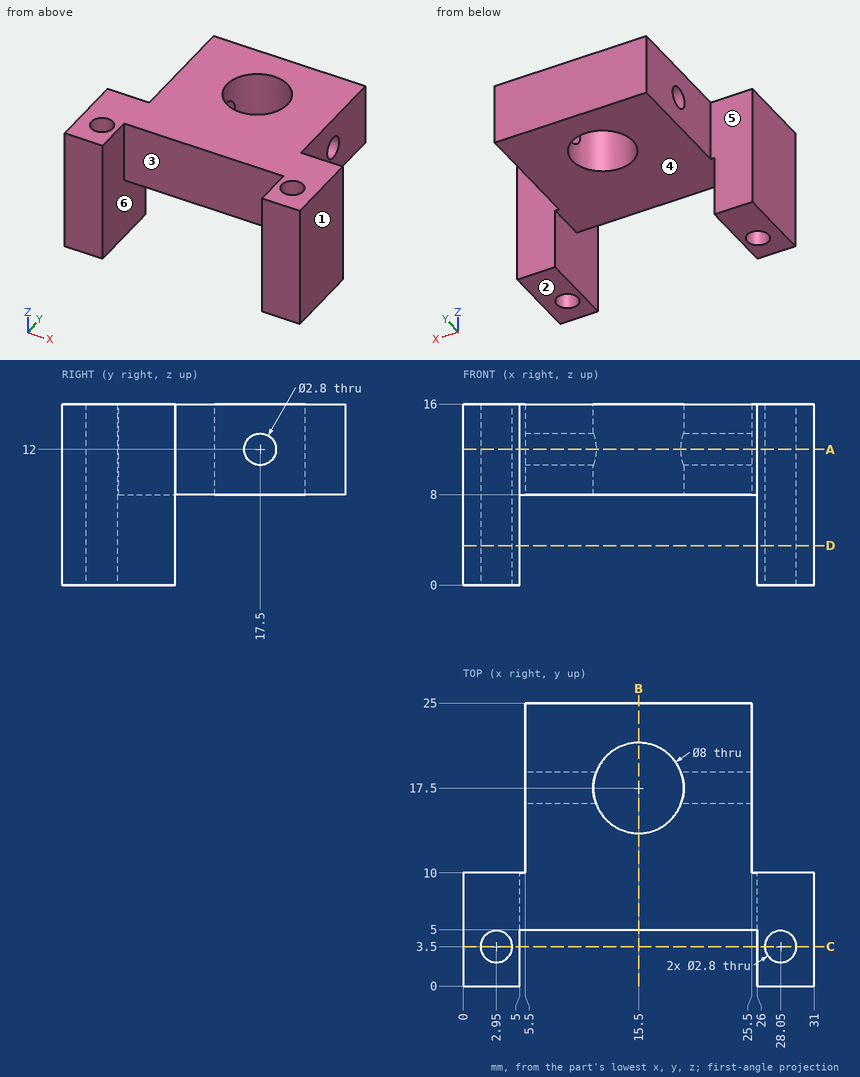
For this review, use the dimensioned drawing (mm, ordinates from the lowest corner) and the shaded views. A direction names the side the tool comes from. Coordinates: 2 decimals unless noted, no trailing zeros. Order: outer loops, then holes, each group sorted by start corner. A loop starts at its lowest first (then second) coordinate and runs counter-clockwise, first axis right, second up. Notation, with made-up numbers: (-16.5, 39.5) -> (37.5, 39.5) arc R10 ccw to (37.5, 48.5) -> close; hole circle Ø8 at (-24, -14.5). An arc over 180 degrees is marked (long way). One line per item, written item: value. Start each with the question number.
Q1. Take a section at B-B, the plane x = 15.5. State the section outline as (y, z) points.
Q2. Take a section at A-A, the plane z = 12. State the section outline as (x, y) points, then the cut area to 3 significant figures.
Q3. Tool access review of the marked faces 4, 5 and 6: name each direction out of +Z, -Z, +X, -X, +Y, -Y from which nothing blocks a thin tool from reaching the whole face with its end or side.
Q4. Insertion check: pin 1 Ø3 at (x, z) = (2.5, 11.5) entering from +Y; pin 2 Ø3 at (x, z) = (12, 12.5) entering from -Y; pin 3 Ø2.5 at (y, z) = (17.5, 11.5) entering from -X. Each pin has a flat end and moves straight along its axis. Give the tip position at first contact, or say it passes through.
Q5. For probe 1 along Y at (x, z) = (24.25, 12); probe 2 along X at (y, z) = (4.5, 12.5); probe 3 along Y at (x, z) = (15.5, 13), list the stretches that pass through material, from the lowest coordinate up.
Q6. Mouldability with a two-part tool opening along X and no side actions: class the marked faces 1, 2 and 3 as pulls with the +X half, pulls with the -X half, needs draft (parallel to the pull), parting line crosses it, or undercut.
Q7. Take a section at D-D, the plane z = 3.5. State the section outline as (x, y) points.
Q8. Take a section at C-C, the plane y = 3.5. State the section outline as (x, z) points, then the cut area to 3 significant figures.
Values follow:
1. outline: (5, 8) -> (13.5, 8) -> (13.5, 16) -> (5, 16) -> close; (21.5, 8) -> (25, 8) -> (25, 16) -> (21.5, 16) -> close
2. outline: (0, 0) -> (5, 0) -> (5, 5) -> (26, 5) -> (26, 0) -> (31, 0) -> (31, 10) -> (25.5, 10) -> (25.5, 16.1) -> (19.25, 16.1) arc R4 cw to (11.75, 16.1) -> (5.5, 16.1) -> (5.5, 10) -> (0, 10) -> close; (5.5, 18.9) -> (11.75, 18.9) arc R4 cw to (19.25, 18.9) -> (25.5, 18.9) -> (25.5, 25) -> (5.5, 25) -> close; hole circle Ø2.8 at (2.95, 3.5); hole circle Ø2.8 at (28.05, 3.5)
2. area: 408 mm2
3. face 4: -Z, +Y, -Y
3. face 5: +Z, -Z, -X, +Y
3. face 6: -Z, -Y
4. pin 1: stops at y = 10
4. pin 2: stops at y = 5
4. pin 3: stops at x = 5.5
5. probe 1: y = 5 to 16.1, 18.9 to 25
5. probe 2: x = 0 to 1.97, 3.93 to 5, 26 to 27.07, 29.03 to 31
5. probe 3: y = 5 to 13.5, 21.5 to 25
6. face 1: pulls with the +X half
6. face 2: needs draft
6. face 3: undercut
7. outline: (0, 0) -> (5, 0) -> (5, 10) -> (0, 10) -> close; (26, 0) -> (31, 0) -> (31, 10) -> (26, 10) -> close; hole circle Ø2.8 at (2.95, 3.5); hole circle Ø2.8 at (28.05, 3.5)
8. outline: (0, 0) -> (1.55, 0) -> (1.55, 16) -> (0, 16) -> close; (4.35, 0) -> (5, 0) -> (5, 16) -> (4.35, 16) -> close; (26, 0) -> (26.65, 0) -> (26.65, 16) -> (26, 16) -> close; (29.45, 0) -> (31, 0) -> (31, 16) -> (29.45, 16) -> close
8. area: 70.4 mm2
